```python
from build123d import *

# Parameters (mm, degrees)
F0_W      = 160
F0_H      = 85
F1_DEPTH  = 2.7
F3_DEPTH  = 1
F4_W      = 8
F4_H      = 8
F5_DEPTH  = 50
F6_DEPTH  = 50
F8_DEPTH  = 2.5
F9_W      = 144
F9_H      = 2.387096
F9_W_2    = 2.1
F9_H_2    = 69
F9_H_3    = 2.1
F10_DEPTH = 9.5


with BuildPart() as f1:
    # F0 (on Top) → F1 (new body)
    with BuildSketch(Plane.XY):
        with Locations((-80, 42.5)):
            Rectangle(F0_W, F0_H)
    extrude(amount=F1_DEPTH)

    # F2 (on face) → F3 (join)
    with BuildSketch(Plane.XY.offset(2.7)):
        Polygon((-1.5, 42.5), (-1.5, 83.5), (-80, 83.5), (-158.5, 83.5), (-158.5, 42.5), (-158.5, 1.5), (-80, 1.5), (-1.5, 1.5), align=None)
    extrude(amount=F3_DEPTH)

    # F4 (on face) → F5 (join)
    with BuildSketch(Plane(origin=(0, 0, 0), x_dir=(1, 0, 0), z_dir=(0, 0, -1))):
        with Locations((-156, -4)):
            Rectangle(F4_W, F4_H)
    extrude(amount=F5_DEPTH)

    # F4 (on face) → F6 (join)
    with BuildSketch(Plane(origin=(0, 0, 0), x_dir=(1, 0, 0), z_dir=(0, 0, -1))):
        with Locations((-156, -4)):
            Rectangle(F4_W, F4_H)
        with Locations((-156, -81)):
            Rectangle(F4_W, F4_H)
        with Locations((-4, -81)):
            Rectangle(F4_W, F4_H)
        with Locations((-4, -4)):
            Rectangle(F4_W, F4_H)
    extrude(amount=F6_DEPTH)

    # F7 (on face) → F8 (join)
    with BuildSketch(Plane.XY.offset(3.7)):
        Polygon((-160, 42.5), (-160, 0), (-80, 0), (0, 0), (0, 42.5), (0, 85), (-80, 85), (-160, 85), align=None)
    extrude(amount=F8_DEPTH)

    # F9 (on face) → F10 (join)
    with BuildSketch(Plane(origin=(0, 0, 0), x_dir=(1, 0, 0), z_dir=(0, 0, -1))):
        with Locations((-80, -1.193548)):
            Rectangle(F9_W, F9_H)
        with Locations((-158.95, -42.5)):
            Rectangle(F9_W_2, F9_H_2)
        with Locations((-1.05, -42.5)):
            Rectangle(F9_W_2, F9_H_2)
        with Locations((-80, -83.95)):
            Rectangle(F9_W, F9_H_3)
    extrude(amount=F10_DEPTH)


solid = f1.part
```
Here's how the part is built. I have some questions about the finished solid (model axes, mm). A direction names the side the tool comes from. Coordinates: 2 decimals unless noted, no trailing zeros. Loops run counter-clockwise (first coordinate to the right, second up) from the corner with the lowest first, then second, coordinate; pieces in that order, holes last. Notation, with made-up numbers: (46.25, -19.75) - (55.25, -19.75) arc R22 ccw to (55.25, -0.75) - close; hole circle Ø8 at (-12.5, 9). An arc over 180 degrees is marked (long way). Return JSON: item names as keys, results as strings. Group by question number.
Item 1: If we section it at A-A on z = -12.5: Write out the boundary of the cut face in (x, y), and give its area (3 significant figures).
Item 2: If we section it at B-B on y = 41: Write out the boundary of the cut face in (x, z), and give its area (3 significant figures).
Item 3: Will these pins go through, and if not, where does the flat tip stop? P1, Ø5, axis at x = -93.5, y = 65, coming from the -Z side; P2, Ø0.7, axis at x = -68, y = 2, coming from the -Z side; P3, Ø0.5, axis at x = -109.5, z = 3, coming from the +Y side.
Item 4: I need wall thicknesses on line 1 (Y direction, x = -116, z = -5); line 2 (X direction, y = 6.5, z = -44.5); line 3 (Z direction, x = -14, y = 20.5). Which ranges of each line are inside material? Lowest first, please. Write a range as from..to.
Item 5: We'd pull the mould along X, two halves only. Please class faces 3 (the face through (-152, 81, -25)), 4 (the face through (-152, 4, -25)), 5 (the face through (-4, 4, -50)), 6 (the face through (0, 42, -6)): +X half, -X half, draft (parallel to the pull), parting line (faces both ways), or undercut.
Item 6: If we section it at D-D on z = -4: Write out the boundary of the cut face in (x, y), and give its area (3 significant figures).
Item 7: On a 3-axis mill with a long thin cutter (end or side, diameter ignored), from which of +Z, -Z, +X, -X, +Y, -Y can I reach the whole of each face in a straight line? I mean faces 1 (the face through (-160, 43, -6)), 2 (the face through (-4, 77, -25)). Say none if no direction works.
Item 8: If we section it at C-C on x = -131: Write out the boundary of the cut face in (y, z), and give its area (3 significant figures).
Calculated:
{
 "1": {"outline": "(-160, 0) - (-152, 0) - (-152, 8) - (-160, 8) - close; (-160, 77) - (-152, 77) - (-152, 85) - (-160, 85) - close; (-8, 0) - (0, 0) - (0, 8) - (-8, 8) - close; (-8, 77) - (0, 77) - (0, 85) - (-8, 85) - close", "area": "256 mm^2"},
 "2": {"outline": "(-160, -9.5) - (-157.9, -9.5) - (-157.9, 0) - (-2.1, 0) - (-2.1, -9.5) - (0, -9.5) - (0, 2.7) - (-1.5, 2.7) - (-1.5, 3.7) - (0, 3.7) - (0, 6.2) - (-160, 6.2) - (-160, 3.7) - (-158.5, 3.7) - (-158.5, 2.7) - (-160, 2.7) - close", "area": "1,030 mm^2"},
 "3": {"P1": "stops at z = 0", "P2": "stops at z = -9.5", "P3": "stops at y = 83.5"},
 "4": {"line 1": "y = 0..2.39, 82.9..85", "line 2": "x = -160..-152, -8..0", "line 3": "z = 0..6.2"},
 "5": {"face 3": "undercut", "face 4": "undercut", "face 5": "draft", "face 6": "+X half"},
 "6": {"outline": "(-160, 0) - (0, 0) - (0, 85) - (-160, 85) - close; hole (-157.9, 8) - (-152, 8) - (-152, 2.39) - (-8, 2.39) - (-8, 8) - (-2.1, 8) - (-2.1, 77) - (-8, 77) - (-8, 82.9) - (-152, 82.9) - (-152, 77) - (-157.9, 77) - close", "area": "1,190 mm^2"},
 "7": {"face 1": "+Z, -Z, -X, +Y, -Y", "face 2": "-Z"},
 "8": {"outline": "(0, -9.5) - (2.39, -9.5) - (2.39, 0) - (82.9, 0) - (82.9, -9.5) - (85, -9.5) - (85, 2.7) - (83.5, 2.7) - (83.5, 3.7) - (85, 3.7) - (85, 6.2) - (0, 6.2) - (0, 3.7) - (1.5, 3.7) - (1.5, 2.7) - (0, 2.7) - close", "area": "567 mm^2"}
}
